from build123d import *

# Parameters (mm, degrees)
F1_DEPTH  = 28
F2_W      = 33
F2_H      = 22
F3_DEPTH  = 33
F6_DEPTH  = 25
F7_DEPTH  = 25
F4_W      = 8
F4_H      = 8
F4_W_2    = 3
F8_DEPTH  = 2
F5_W      = 32
F5_H      = 3
F9_DEPTH  = 2
F9_TAPER  = 20
F5_W_2    = 3
F5_H_2    = 8
F5_W_3    = 8
F10_DEPTH = 2
F4_W_3    = 32
F4_H_2    = 3
F11_DEPTH = 2
F11_TAPER = 20
F12_SIZE  = 1
F13_SIZE  = 0.5
F14_SIZE  = 4


with BuildPart() as f1:
    # F0 (on Top) → F1 (new body)
    with BuildSketch(Plane.XY):
        Polygon((-19, -19), (19, -19), (19, -13), (-13, 19), (-19, 19), align=None)
    extrude(amount=F1_DEPTH)

    # F2 (on face) → F3 (cut, through all)
    with BuildSketch(Plane.YZ.offset(19)):
        with Locations((2.5, 14)):
            Rectangle(F2_W, F2_H)
    extrude(amount=-F3_DEPTH, mode=Mode.SUBTRACT)

    # F4 (on face) → F6 (cut)
    with BuildSketch(Plane.XZ.offset(19)):
        with BuildLine():
            Line((-1, 11.25), (7, 11.25))
            ThreePointArc((7, 11.25), (9.75, 14), (7, 16.75))
            Line((7, 16.75), (-1, 16.75))
            ThreePointArc((-1, 16.75), (-3.75, 14), (-1, 11.25))
        make_face()
    extrude(amount=-F6_DEPTH, mode=Mode.SUBTRACT)

    # F5 (on face) → F7 (cut)
    with BuildSketch(Plane(origin=(-19, 0, 0), x_dir=(0, -1, 0), z_dir=(-1, 0, 0))):
        with BuildLine():
            Line((-7, 11.25), (1, 11.25))
            ThreePointArc((1, 11.25), (3.75, 14), (1, 16.75))
            Line((1, 16.75), (-7, 16.75))
            ThreePointArc((-7, 16.75), (-9.75, 14), (-7, 11.25))
        make_face()
    extrude(amount=-F7_DEPTH, mode=Mode.SUBTRACT)

    # F4 (on face) → F8 (join)
    with BuildSketch(Plane.XZ.offset(19)):
        with Locations((-12, 14)):
            Rectangle(F4_W, F4_H)
        with Locations((14.5, 14)):
            Rectangle(F4_W_2, F4_H)
    extrude(amount=F8_DEPTH)

    # F5 (on face) → F9 (cut)
    with BuildSketch(Plane(origin=(-19, 0, 0), x_dir=(0, -1, 0), z_dir=(-1, 0, 0))):
        with Locations((0, 23)):
            Rectangle(F5_W, F5_H)
        with Locations((0, 5)):
            Rectangle(F5_W, F5_H)
    extrude(amount=-F9_DEPTH, taper=F9_TAPER, mode=Mode.SUBTRACT)

    # F5 (on face) → F10 (join)
    with BuildSketch(Plane(origin=(-19, 0, 0), x_dir=(0, -1, 0), z_dir=(-1, 0, 0))):
        with Locations((-14.5, 14)):
            Rectangle(F5_W_2, F5_H_2)
        with Locations((12, 14)):
            Rectangle(F5_W_3, F5_H_2)
    extrude(amount=F10_DEPTH)

    # F4 (on face) → F11 (cut)
    with BuildSketch(Plane.XZ.offset(19)):
        with Locations((0, 23)):
            Rectangle(F4_W_3, F4_H_2)
        with Locations((0, 5)):
            Rectangle(F4_W_3, F4_H_2)
    extrude(amount=-F11_DEPTH, taper=F11_TAPER, mode=Mode.SUBTRACT)

    # F12
    f12_edges = [f1.edges().sort_by_distance(p)[0] for p in [
        (-19, -19, 14),
        (19, -19, 14),
        (-19, 19, 14),
    ]]
    chamfer(f12_edges, length=F12_SIZE)

    # F13
    f13_edges = [f1.edges().sort_by_distance(p)[0] for p in [
        (-21, 14.5, 10),
        (-21, 13, 14),
        (-21, 14.5, 18),
        (-21, 16, 14),
        (-21, -12, 10),
        (-21, -16, 14),
        (-21, -12, 18),
        (-21, -8, 14),
        (-12, -21, 10),
        (-8, -21, 14),
        (-12, -21, 18),
        (-16, -21, 14),
        (14.5, -21, 10),
        (16, -21, 14),
        (14.5, -21, 18),
        (13, -21, 14),
        (-19, 13, 14),
        (-19, -16, 14),
        (-16, -19, 14),
        (13, -19, 14),
        (-19, -8, 14),
        (-19, 16, 14),
        (16, -19, 14),
        (-8, -19, 14),
    ]]
    chamfer(f13_edges, length=F13_SIZE)

    # F14
    f14_edges = [f1.edges().sort_by_distance(p)[0] for p in [
        (-14, 2.5, 3),
        (2.5, -14, 3),
        (-14, 2.5, 25),
        (2.5, -14, 25),
        (-14, -14, 14),
    ]]
    chamfer(f14_edges, length=F14_SIZE)


solid = f1.part
Could you check a few things on this model? Use its own coordinates, in mm. A direction names the side the tool comes from. Give positions to 0.01 mm unless a question says otherwise; leave off trailing zeros. Order: outer loops, then holes, each group sorted by start corner. A loop starts at its lowest first (then second) coordinate and runs counter-clockwise, first axis right, second up.
Item 1: If we section it at A-A, the plane z = 26.25: Write out the boundary of the cut face in (x, y).
Item 2: For faces 4 (the face through (-20, 16, 14)), 5 (the face through (-20, -8, 14)), 6 (the face through (13, -20, 14)), 7 (the face through (-12, -12, 14)), which set-ups out of +Z, -Z, +X, -X, +Y, -Y let a thin tool reach every point of the face, with its end or its side?
Item 3: I'm going to push flat-ended pins straight in: pin 1 (10 mm diameter, centred on x = -9.5, z = 17, fed in from +Y); pin 2 (0.8 mm diameter, centred on x = -19.5, y = 15, fed in from -Z); pin 3 (1.1 mm diameter, centred on x = -20, z = 15, fed in from +Y); pin 4 (10 mm diameter, centred on y = 3.5, z = 7.5, fed in from +X). Where does each tip first touch, or does it pass through?
Item 4: I need wall thicknesses on line 1 (Z direction, x = 6, y = -4); line 2 (Z direction, x = -16, y = 6); line 3 (Z direction, x = -18.5, y = 4.5). Which ranges of each line are inside material? Lowest first, please.
Item 5: If we mould it in two halves opening along Y, with no side actions, what happens to faces 1 (the face through (-16.54, -3.75, 13.94)), 2 (the face through (-3, -3, 3)), 3 (the face through (5, -12, 5))? For each: pulls with the +Y half, pulls with the -Y half, needs draft (parallel to the pull), parting line crosses it, or undercut.
Item 6: If we section it at B-B, the plane z = 14: Count the separate pieces of the cut face and the enclosed holes in it, plus the area to 4 significant figures.
Values:
1. outline: (-19, -18) - (-18, -19) - (18, -19) - (19, -18) - (19, -13) - (-13, 19) - (-18, 19) - (-19, 18) - close
2. face 4: +Z, -Z, -X, +Y
2. face 5: +Z, -Z, -X
2. face 6: +Z, -Z, -Y
2. face 7: +X, +Y
3. pin 1: stops at y = 19
3. pin 2: stops at z = 10
3. pin 3: stops at y = 16.05
3. pin 4: stops at x = 4.68
4. line 1: z = 0 to 3, 25 to 28
4. line 2: z = 0 to 11.25, 16.75 to 28
4. line 3: z = 0 to 3.68, 6.32 to 11.25, 16.75 to 21.68, 24.32 to 28
5. face 1: undercut
5. face 2: needs draft
5. face 3: pulls with the +Y half
6. separate pieces: 3
6. enclosed holes: 0
6. area: 270.5 mm2
